```python
from build123d import *

# Parameters (mm, degrees)
SKETCH2_W           = 4.24
SKETCH2_H           = 4.24
BOSS_EXTRUDE1_DEPTH = 5


with BuildPart() as part:
    # Sketch2 → Boss-Extrude1 (new body)
    with BuildSketch(Plane(origin=(0, 0, 0), x_dir=(1, 0, 0), z_dir=(0, 1, 0))):
        with BuildLine():
            Line((7.711630813, -9.356936378), (4.247529198, -11.356936378))
            Line((4.247529198, -11.356936378), (2.659936491, -9.607145147))
            Line((2.659936491, -9.607145147), (2.419219348, -9.341834817))
            ThreePointArc((2.419219348, -9.341834817), (0, -9.65), (-2.419219348, -9.341834817))
            Line((-2.419219348, -9.341834817), (-2.659936491, -9.607145147))
            Line((-2.659936491, -9.607145147), (-4.247529198, -11.356936378))
            Line((-4.247529198, -11.356936378), (-7.711630813, -9.356936378))
            Line((-7.711630813, -9.356936378), (-6.990063509, -7.107145147))
            Line((-6.990063509, -7.107145147), (-6.880656595, -6.766022821))
            ThreePointArc((-6.880656595, -6.766022821), (-8.357145147, -4.825), (-9.299875943, -2.575811995))
            Line((-9.299875943, -2.575811995), (-9.65, -2.5))
            Line((-9.65, -2.5), (-11.959160012, -2))
            Line((-11.959160012, -2), (-11.959160012, 2))
            Line((-11.959160012, 2), (-9.65, 2.5))
            Line((-9.65, 2.5), (-9.299875943, 2.575811995))
            ThreePointArc((-9.299875943, 2.575811995), (-8.357145147, 4.825), (-6.880656595, 6.766022821))
            Line((-6.880656595, 6.766022821), (-6.990063509, 7.107145147))
            Line((-6.990063509, 7.107145147), (-7.711630813, 9.356936378))
            Line((-7.711630813, 9.356936378), (-4.247529198, 11.356936378))
            Line((-4.247529198, 11.356936378), (-2.659936491, 9.607145147))
            Line((-2.659936491, 9.607145147), (-2.419219348, 9.341834817))
            ThreePointArc((-2.419219348, 9.341834817), (0, 9.65), (2.419219348, 9.341834817))
            Line((2.419219348, 9.341834817), (2.659936491, 9.607145147))
            Line((2.659936491, 9.607145147), (4.247529198, 11.356936378))
            Line((4.247529198, 11.356936378), (7.711630813, 9.356936378))
            Line((7.711630813, 9.356936378), (6.990063509, 7.107145147))
            Line((6.990063509, 7.107145147), (6.880656595, 6.766022821))
            ThreePointArc((6.880656595, 6.766022821), (8.357145147, 4.825), (9.299875943, 2.575811995))
            Line((9.299875943, 2.575811995), (9.65, 2.5))
            Line((9.65, 2.5), (11.959160012, 2))
            Line((11.959160012, 2), (11.959160012, -2))
            Line((11.959160012, -2), (9.65, -2.5))
            Line((9.65, -2.5), (9.299875943, -2.575811995))
            ThreePointArc((9.299875943, -2.575811995), (8.357145147, -4.825), (6.880656595, -6.766022821))
            Line((6.880656595, -6.766022821), (6.990063509, -7.107145147))
            Line((6.990063509, -7.107145147), (7.711630813, -9.356936378))
        make_face()
        Rectangle(SKETCH2_W, SKETCH2_H, mode=Mode.SUBTRACT)
    extrude(amount=BOSS_EXTRUDE1_DEPTH)


solid = part.part
```
The listing builds one solid part. Answer for the finished solid, in the listing's coordinates (mm). A direction names the side the tool comes from. Round coordinates to 2 decimals unless told otherwise and drop trailing zeros. Loops run counter-clockwise (first coordinate to the right, second up) from the corner with the lowest first, then second, coordinate; pieces in that order, holes last. Notation, with made-up numbers: (75, -6.75) - (120, -6.75) arc R13 cw to (120, 13.25) - close; hole circle Ø10 at (-34, -27.5). An arc over 180 degrees is marked (long way). Return JSON: item names as keys, results as strings. Group by question number.
1. The mould has two halves that part along Z. Classify faces 4 (the flat face through (0, 2, 2.12)), 5 (the cylindrical face through (-0.03, 2.46, -9.65)), 6 (the cylindrical face through (0.03, 2.46, 9.65)): pulls with the +Z half, pulls with the -Z half, needs draft (parallel to the pull), parting line crosses it, or undercut.
2. The part is cut by section B-B on x = 3.25. Determine the outline of the cut face in (y, z), then the cut area to 3 significant figures.
3. Which of the six approach directions +Z, -Z, +X, -X, +Y, -Y give full straight-line access (tool end or side, diameter ignored) to faces 1 (the cylindrical face through (8.34, 2.465, -4.855)), 2 (the cylindrical face through (-8.34, 2.465, 4.855)), 3 (the flat face through (0, 2, -2.12))?
4. Each of these flat-tipped pins is pushed along its axis until it touches: P1, Ø1.3, axis at x = 1, y = 3, coming from the +Z side; P2, Ø1.5, axis at x = -6.5, y = 3.5, coming from the -Z side; P3, Ø3, axis at x = 2.5, y = 4, coming from the +Z side. Where does it stop, or does it pass through?
5. Consider probe 1 along X at (y, z) = (0.5, 1.75); probe 2 along X at (y, z) = (4.5, 10); probe 3 along Z at (x, y) = (1.5, 0.35). Determine where each line is inside the solid, lowest interval first.
6. The part is cut by section C-C on z = -4.75. Determine the outline of the cut face in (x, y).
7. The part is cut by section A-A on z = 1.5. Determine the outline of the cut face in (x, y).
Resolved:
{
 "1": {"face 4": "undercut", "face 5": "pulls with the -Z half", "face 6": "pulls with the +Z half"},
 "2": {"outline": "(0, -10.26) - (5, -10.26) - (5, 10.26) - (0, 10.26) - close", "area": "103 mm²"},
 "3": {"face 1": "+X, +Y, -Y", "face 2": "-X, +Y, -Y", "face 3": "+Y, -Y"},
 "4": {"P1": "stops at z = 9.64", "P2": "stops at z = -10.49", "P3": "stops at z = 11.08"},
 "5": {"probe 1": "x = -11.96 to -2.12, 2.12 to 11.96", "probe 2": "x = -6.6 to -3.02, 3.02 to 6.6", "probe 3": "z = -9.53 to -2.12, 2.12 to 9.53"},
 "6": {"outline": "(-8.4, 0) - (8.4, 0) - (8.4, 5) - (-8.4, 5) - close"},
 "7": {"outline": "(-11.96, 0) - (-2.12, 0) - (-2.12, 5) - (-11.96, 5) - close; (2.12, 0) - (11.96, 0) - (11.96, 5) - (2.12, 5) - close"}
}
